Check sheet for the modelled part. Datum: model origin and axes. Units: mm. A direction names the side the tool comes from. Coordinates: 2 decimals unless noted, no trailing zeros. Loops run counter-clockwise (first coordinate to the right, second up) from the corner with the lowest first, then second, coordinate; pieces in that order, holes last. Notation, with made-up numbers: (39, 62) -> (91, 62) arc R21 ccw to (91, 78) -> close; hole circle Ø11 at (86.25, 65). An arc over 180 degrees is marked (long way). Use one line per item in the form item = value.
from build123d import *

# Parameters (mm, degrees)
ESQUISSE1_W                = 96
ESQUISSE1_H                = 30
BOSS_EXTRU_1_DEPTH         = 21
ESQUISSE2_W                = 7.5
ESQUISSE2_H                = 15
ESQUISSE2_W_2              = 2
ESQUISSE2_H_2              = 12
ENL_V_MAT_EXTRU_1_DEPTH    = 12
R_P_TITION_LIN_AIRE1_COUNT = 4
R_P_TITION_LIN_AIRE1_PITCH = 17.5


with BuildPart() as part:
    # Esquisse1 → Boss.-Extru.1 (new body)
    with BuildSketch(Plane.XY):
        with Locations((14.064055763, -0.233160622)):
            Rectangle(ESQUISSE1_W, ESQUISSE1_H)
    extrude(amount=BOSS_EXTRU_1_DEPTH)

    # Esquisse2 → Enlèv. mat.-Extru.1 (cut)
    with BuildSketch(Plane.XY.offset(21)):
        with Locations((-15.185944237, -0.233160622)):
            Rectangle(ESQUISSE2_W, ESQUISSE2_H)
        with Locations((-14.185944237, -0.233160622)):
            Rectangle(ESQUISSE2_W_2, ESQUISSE2_H_2, mode=Mode.SUBTRACT)
    enl_v_mat_extru_1 = extrude(amount=-ENL_V_MAT_EXTRU_1_DEPTH, mode=Mode.SUBTRACT)

    # Répétition linéaire1: Enlèv. mat.-Extru.1 ×4
    with Locations(*[(i * R_P_TITION_LIN_AIRE1_PITCH, 0, 0) for i in range(1, R_P_TITION_LIN_AIRE1_COUNT)]):
        add(enl_v_mat_extru_1, mode=Mode.SUBTRACT)


solid = part.part
(1) Section check B-B, the plane x = 18. Record the boundary of the cut face in (y, z), plus the area to 3 significant figures.
Established:
outline = (-15.23, 0) -> (14.77, 0) -> (14.77, 21) -> (7.27, 21) -> (7.27, 9) -> (-7.73, 9) -> (-7.73, 21) -> (-15.23, 21) -> close
area = 450 mm²
(2) Go/stop test with a flat-tipped pin: P1, Ø3, axis at x = 45, y = 4.5, coming from the -Z side. Record where the tip stops, or that it passes through.
Established:
P1 = 0
(3) Tool access check on faces 1 (the flat face through (39.314, 0, 15)), 2 (the flat face through (38, 0, 21)). Record the directions out of +Z, -Z, +X, -X, +Y, -Y that give a thin tool (end or side, any length) a straight path to the whole face; none if there is none.
Established:
face_1 = +Z
face_2 = +Z, +X, -X, +Y, -Y
(4) Scan lines: line 1 along X through (y, z) = (7, 19); line 2 along Y through (x, z) = (37, 11); line 3 along Z through (x, y) = (-15.5, 6.5). Record each from-to range of solid material in increasing order.
Established:
line_1 = -33.94 to -18.94, -11.44 to -1.44, 6.06 to 16.06, 23.56 to 33.56, 41.06 to 62.06
line_2 = -15.23 to -7.73, 7.27 to 14.77
line_3 = 0 to 9
(5) Section check A-A, the plane z = 12.5. Give the number of separate pieces and of enclosed holes in the cut face, plus the area to 3 significant figures.
Established:
separate_pieces = 5
enclosed_holes = 4
area = 2,530 mm²
(6) Mould release check, pull along X, two halves, no side actions. Record for faces 3 (the flat face through (13, -15.233, 10)), 4 (the flat face through (21, 5.767, 15)): +X half, -X half, draft (parallel to the pull), parting line (faces both ways), or undercut.
Established:
face_3 = draft
face_4 = undercut
